Can you work these out from the model? Positions are in its coordinate system, mm. A direction names the side the tool comes from. Give positions to 0.01 mm unless a question says otherwise; leave off trailing zeros. Write each loop counter-clockwise with the first axis right and the second up, starting at its lowest first coordinate (ties: lowest second). Pieces come first, ordered by that corner, then holes. Notation, with made-up numbers: (-39, 22) - (-20, 22) arc R31 cw to (-20, 50) - close; hole circle Ø7 at (-23, 23.25). An arc over 180 degrees is marked (long way). Use a Markdown table: item, result. Add a question column.
```python
from build123d import *

# Parameters (mm, degrees)
SWEEP4_PROFILE_R = 0.6


with BuildPart() as part:
    # Sweep4: sweep along a path in Sketch4
    with BuildLine(Plane(origin=(0, 0, 0), x_dir=(0, 0, -1), z_dir=(1, 0, 0))) as sweep4_path:
        Line((0, 0), (0, 8))
        ThreePointArc((0, 8), (-0.292893219, 8.707106781), (-1, 9))
        Line((-1, 9), (-43.85922, 9))
        ThreePointArc((-43.85922, 9), (-44.566326781, 8.707106781), (-44.85922, 8))
        Line((-44.85922, 8), (-44.85922, 0))
    # Sweep4 profile (on start of the path) → Sweep4 (sweep)
    with BuildSketch(Plane.ZX):
        Circle(SWEEP4_PROFILE_R)
    sweep(path=sweep4_path.line)


solid = part.part
```
Q1. On a 3-axis mill with a long thin cutter (end or side, diameter ignored), from which of +Z, -Z, +X, -X, +Y, -Y can I reach the whole of each face in a straight line? I mean faces 3 (the cylindrical face through (0.506, 4.056, 0.323)), 4 (the flat face through (0, 0, 0)). Say none if no direction works.
Q2. Suppose I cut it at C-C (z = 41). Please give me the cut outline in (x, y), and give its area (3 significant figures).
Q3. Suppose I cut it at B-B (x = -0.25). Please give me the cut outline in (y, z).
Q4. Suppose I cut it at A-A (y = 6). Please give me the cut outline in (x, z), and give its area (3 significant figures).
Q5. If we mould it in two halves opening along Z, with no side actions, what happens to faces 1 (the cylindrical face through (0, 9.6, 22.7)), 2 (the flat face through (0, 0, 45))? For each: released by +Z, released by -Z, zero draft, split by the parting line, or undercut.
Q6. I'm going to push a flat-ended pin straight in: P1, Ø4, axis at y = 7, z = 13.5, coming from the -X side. Where does the tip first touch, or does it pass through?
Q7. If I drill on probe 1 along Z at (x, y) = (0.1, 5.25); probe 2 along Y at (x, z) = (-0.1, 33); probe 3 along Z at (x, y) = (0.3, 6), over which ranges is the centre line in solid material (lowest first)? Write a range as [from, to].
Derived:
| question | item | result |
|---|---|---|
| 1 | face 3 | -Y |
| 1 | face 4 | +Z, -Z, +X, -X, -Y |
| 2 | outline | circle Ø1.2 at (0, 9) |
| 2 | area | 1.13 mm² |
| 3 | outline | (0, -0.55) - (8, -0.55) arc R1.55 ccw to (9.55, 1) - (9.55, 43.86) arc R1.55 ccw to (8, 45.4) - (0, 45.4) - (0, 44.31) - (8, 44.31) arc R0.45 cw to (8.45, 43.86) - (8.45, 1) arc R0.45 cw to (8, 0.55) - (0, 0.55) - close |
| 4 | outline | circle Ø1.2 at (0, 0); circle Ø1.2 at (0, 44.86) |
| 4 | area | 2.26 mm² |
| 5 | face 1 | undercut |
| 5 | face 2 | zero draft |
| 6 | P1 | x = -0.6 |
| 7 | probe 1 | [-0.59, 0.59], [44.27, 45.45] |
| 7 | probe 2 | [8.41, 9.59] |
| 7 | probe 3 | [-0.52, 0.52], [44.34, 45.38] |
